Geometry: final body of the model. Coordinates: model frame, mm. Give positions to 0.01 mm unless a question says otherwise; leave off trailing zeros. Write each loop counter-clockwise with the first axis right and the second up, starting at its lowest first coordinate (ties: lowest second). Pieces come first, ordered by that corner, then holes. Notation, with made-up numbers: (27, 75.25) -> (31, 75.25) arc R15 cw to (31, 91.25) -> close; hole circle Ø6 at (27, 30). An arc over 180 degrees is marked (long way). Answer in a Markdown table with one row per item. Add a question column.
Item 1: Section query D-D on x = 18.5. Output: boundary loops of the cut face in (y, z), plus the area to 3 significant figures.
Item 2: Section query C-C on z = 1.5. Output: boundary loops of the cut face in (x, y).
Item 3: Material intervals for probe 1 along Y at (x, z) = (0, -0.45); probe 2 along X at (y, z) = (2.5, 0.05); probe 3 along X at (y, z) = (16, 1.35), sorted ascending. Write a range as from..to.
Item 4: First-contact query: P1, Ø1, axis at y = -2, z = 1, coming from the -X side. Flat tip, straight axial feed; report the tip coordinate or a pass-through.
Item 5: Section query A-A on y = 0. Output: boundary loops of the cut face in (x, z).
```python
from build123d import *

# Parameters (mm, degrees)
SKETCH1_R           = 22.5
SKETCH1_R_2         = 17.5
BOSS_EXTRUDE1_DEPTH = 2
BOSS_EXTRUDE2_START = 1
SKETCH2_R           = 22.5
BOSS_EXTRUDE2_DEPTH = 1
CUT_EXTRUDE1_START  = -1
SKETCH3_R           = 17.5
CUT_EXTRUDE1_DEPTH  = 1


with BuildPart() as part:
    # Sketch1 → Boss-Extrude1 (new body)
    with BuildSketch(Plane.XY):
        Circle(SKETCH1_R)
        Circle(SKETCH1_R_2, mode=Mode.SUBTRACT)
    extrude(amount=BOSS_EXTRUDE1_DEPTH)

    # Sketch2 → Boss-Extrude2 (add)
    with BuildSketch(Plane(origin=(0, 0, 0), x_dir=(-1, 0, 0), z_dir=(0, 0, -1)).offset(BOSS_EXTRUDE2_START)):
        Circle(SKETCH2_R)
    extrude(amount=-BOSS_EXTRUDE2_DEPTH)

    # Sketch3 → Cut-Extrude1 (cut)
    with BuildSketch(Plane.XY.offset(CUT_EXTRUDE1_START)):
        Circle(SKETCH3_R)
    extrude(amount=CUT_EXTRUDE1_DEPTH, mode=Mode.SUBTRACT)


solid = part.part
```
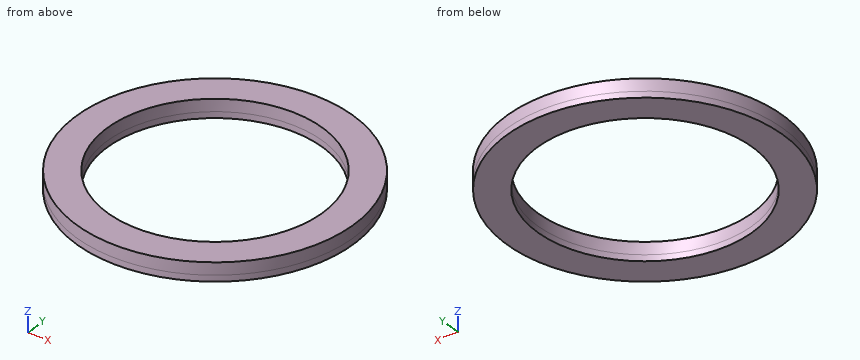
Findings below:
| question | item | result |
|---|---|---|
| 1 | outline | (-12.81, -1) -> (12.81, -1) -> (12.81, 2) -> (-12.81, 2) -> close |
| 1 | area | 76.8 mm^2 |
| 2 | outline | circle Ø45 at (0, 0); hole circle Ø35 at (0, 0) |
| 3 | probe 1 | y = -22.5..-17.5, 17.5..22.5 |
| 3 | probe 2 | x = -22.36..-17.32, 17.32..22.36 |
| 3 | probe 3 | x = -15.82..-7.09, 7.09..15.82 |
| 4 | P1 | stops at x = -22.45 |
| 5 | outline | (-22.5, -1) -> (-17.5, -1) -> (-17.5, 2) -> (-22.5, 2) -> close; (17.5, -1) -> (22.5, -1) -> (22.5, 2) -> (17.5, 2) -> close |
